Drawing for the job (mm, zero at the part's lowest x, y, z). Round coordinates to 2 decimals unless told otherwise and drop trailing zeros. Write each loop counter-clockwise with the first axis right and the second up, starting at its lowest first coordinate (ties: lowest second). Pieces come first, ordered by that corner, then holes. Notation, with made-up numbers: M -38.75,-0.5 L -8.75,-0.5 A18 ccw -8.75,9.5 Z; hole C 32,-5.5 d7. An arc over 180 degrees is marked long. Use a Markdown table: item, result.
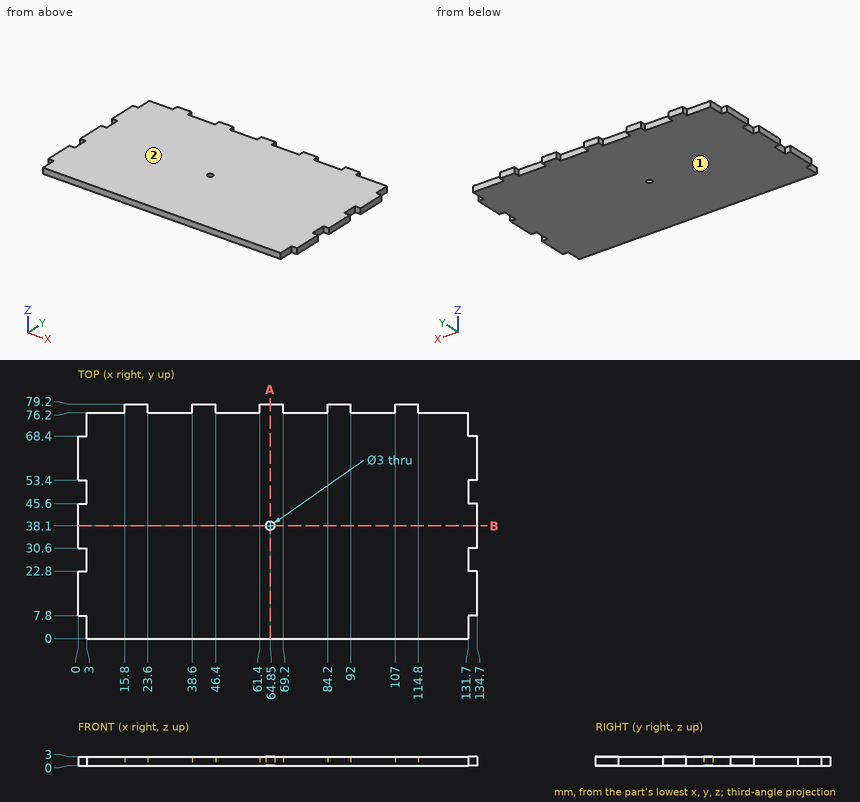
Q1. Drill centre lines: L1, parallel to Y at x = 64.85, z = 0.85; L2, parallel to Y at x = 58.5, z = 0.4; L3, parallel to X at y = 71, z = 2.85. Where is each one in solid material? Low to high.
Response values:
| item | result |
|---|---|
| L1 | y = 0 to 36.6, 39.6 to 79.2 |
| L2 | y = 0 to 76.2 |
| L3 | x = 3 to 131.7 |
Q2. Cut at A-A on x = 64.85. Give the cut face in (y, z), and give its area (3 significant figures).
Response values:
| item | result |
|---|---|
| outline | M 0,0 L 36.6,0 L 36.6,3 L 0,3 Z; M 39.6,0 L 79.2,0 L 79.2,3 L 39.6,3 Z |
| area | 229 mm2 |
Q3. Drop flat-ended pins along their axis: P1, Ø4, axis at x = 64.5, y = 49.5, coming from the -Z side; P2, Ø1.5, axis at y = 78.5, z = 1.5, coming from the -X side; P3, Ø1.5, axis at y = 77.5, z = 1.5, coming from the +X side; P4, Ø0.9, axis at x = 98.5, z = 1, coming from the +Y side. Give the stop position or say it passes through.
Response values:
| item | result |
|---|---|
| P1 | stops at z = 0 |
| P2 | stops at x = 15.8 |
| P3 | stops at x = 114.8 |
| P4 | stops at y = 76.2 |
Q4. Cut at B-B on y = 38.1. Give the cut face in (x, z).
Response values:
| item | result |
|---|---|
| outline | M 0,0 L 63.35,0 L 63.35,3 L 0,3 Z; M 66.35,0 L 134.7,0 L 134.7,3 L 66.35,3 Z |
Q5. Two-plate mould, pull along Z, no slides. Class the marked faces 1 and 2: +Z half, -Z half, draft (parallel to the pull), parting line (faces both ways), or undercut.
Response values:
| item | result |
|---|---|
| face 1 | -Z half |
| face 2 | +Z half |
